Verification items for the finished model (mm, model axes). A direction names the side the tool comes from. Coordinates: 2 decimals unless noted, no trailing zeros. Loops run counter-clockwise (first coordinate to the right, second up) from the corner with the lowest first, then second, coordinate; pieces in that order, holes last.
Q1. Sectioned sample at B-B (z = 1.25). Count the separate pieces of the cut face and the enclosed holes in it, then the cut area to 3 significant figures.
Q2. Sectioned sample at A-A (y = 12.7). Enter the section's corners in (x, z).
Q3. Mould release check, pull along Y, two halves, no side actions. Record for faces 4 (the face through (-26.275, 12.83, 3.026)), 5 (the face through (0, -7, 6.35)), 6 (the face through (-1, -44.069, 3)): +Y half, -Y half, draft (parallel to the pull), parting line (faces both ways), or undercut.
Q4. Access from +Z, -Z, +X, -X, +Y, -Y to the whole of each face (thin tool, end or side, straight path). Record for faces 1 (the face through (15.594, -12.586, 6.162)), 2 (the face through (15.213, -12.806, 3.026)), 3 (the face through (-0.4, 19.2, 6.35)).
Q5. Sectioned sample at C-C (x = -23.5). Enter the section's corners in (y, z), then the cut area to 3 significant figures.
Q6. Go/stop test with flat-tipped pins: P1, Ø2.5, axis at x = -52.39, y = -39.69, coming from the -Z side; P2, Ø6.5, axis at x = -10, y = 15.5, coming from the +Z side. Record where each tip stops, or that it passes through.
Q7. Material ranges on probe 1 along Y at (x, z) = (10, 4); probe 2 along Y at (x, z) = (13.5, 1.25); probe 3 along X at (y, z) = (-17.5, 6.25), recorded low to high.
```python
from build123d import *

# Parameters (mm, degrees)
SKETCH1_W                 = 113.538
SKETCH1_H                 = 88.138
EXTRUDE1_DEPTH            = 6.35
F_8_CLEARANCE_HOLE1_D     = 4.0386
F_8_CLEARANCE_HOLE1_DEPTH = 6.35
FILLET2_R                 = 3.175
SKETCH8_W                 = 40.6908
SKETCH8_H                 = 12.6238
SKETCH8_W_2               = 20.7772
SKETCH8_H_2               = 10.414
CUT_EXTRUDE1_DEPTH        = 0.381
CUT_EXTRUDE2_DEPTH        = 7.35
CUT_EXTRUDE3_DEPTH        = 0.254


with BuildPart() as part:
    # Sketch1 → Extrude1 (new body)
    with BuildSketch(Plane.XY):
        Rectangle(SKETCH1_W, SKETCH1_H)
    extrude(amount=EXTRUDE1_DEPTH)

    # #8 Clearance Hole1
    with Locations(Plane(origin=(-52.3875, 39.6875, 6.35), x_dir=(1, 0, 0), z_dir=(0, 0, 1))):
        with Locations((0, 0), (104.775, 0), (104.775, -79.375), (0, -79.375)):
            Hole(F_8_CLEARANCE_HOLE1_D / 2, depth=F_8_CLEARANCE_HOLE1_DEPTH)

    # Fillet2
    fillet2_edges = [part.edges().sort_by_distance(p)[0] for p in [
        (-56.769, 44.069, 3.175),
        (56.769, 44.069, 3.175),
        (56.769, -44.069, 3.175),
        (-56.769, -44.069, 3.175),
    ]]
    fillet(fillet2_edges, radius=FILLET2_R)

    # Sketch8 → Cut-Extrude1 (cut)
    with BuildSketch(Plane.XY.offset(6.35)):
        with BuildLine():
            ThreePointArc((-20.3454, 6.3881), (-26.6573, 12.7), (-20.3454, 19.0119))
            Line((-20.3454, 19.0119), (-20.3454, 6.3881))
        make_face()
        with Locations((0, 12.7)):
            Rectangle(SKETCH8_W, SKETCH8_H)
        with BuildLine():
            ThreePointArc((20.3454, 19.0119), (26.6573, 12.7), (20.3454, 6.3881))
            Line((20.3454, 6.3881), (20.3454, 19.0119))
        make_face()
        with BuildLine():
            ThreePointArc((10.3886, -7.493), (15.5956, -12.7), (10.3886, -17.907))
            Line((10.3886, -17.907), (10.3886, -7.493))
        make_face()
        with Locations((0, -12.7)):
            Rectangle(SKETCH8_W_2, SKETCH8_H_2)
        with BuildLine():
            Line((-10.3886, -17.907), (-10.3886, -7.493))
            ThreePointArc((-10.3886, -7.493), (-15.5956, -12.7), (-10.3886, -17.907))
        make_face()
    extrude(amount=-CUT_EXTRUDE1_DEPTH, mode=Mode.SUBTRACT)

    # Sketch9 → Cut-Extrude2 (cut, through all)
    with BuildSketch(Plane.XY.offset(6.35)):
        with BuildLine():
            Line((-20.3454, 6.7691), (20.3454, 6.7691))
            ThreePointArc((20.3454, 6.7691), (26.2763, 12.7), (20.3454, 18.6309))
            Line((20.3454, 18.6309), (-20.3454, 18.6309))
            ThreePointArc((-20.3454, 18.6309), (-26.2763, 12.7), (-20.3454, 6.7691))
        make_face()
        with BuildLine():
            Line((10.3886, -7.874), (-10.3886, -7.874))
            ThreePointArc((-10.3886, -7.874), (-15.2146, -12.7), (-10.3886, -17.526))
            Line((-10.3886, -17.526), (10.3886, -17.526))
            ThreePointArc((10.3886, -17.526), (15.2146, -12.7), (10.3886, -7.874))
        make_face()
    extrude(amount=-CUT_EXTRUDE2_DEPTH, mode=Mode.SUBTRACT)

    # Sketch10 → Cut-Extrude3 (cut)
    with BuildSketch(Plane.XY.offset(6.35)):
        with BuildLine():
            Line((20.3454, 2.9591), (-20.3454, 2.9591))
            ThreePointArc((-20.3454, 2.9591), (-30.0863, 12.7), (-20.3454, 22.4409))
            Line((-20.3454, 22.4409), (20.3454, 22.4409))
            ThreePointArc((20.3454, 22.4409), (30.0863, 12.7), (20.3454, 2.9591))
        make_face()
        with BuildLine():
            ThreePointArc((20.3454, 3.2131), (29.8323, 12.7), (20.3454, 22.1869))
            Line((20.3454, 22.1869), (-20.3454, 22.1869))
            ThreePointArc((-20.3454, 22.1869), (-29.8323, 12.7), (-20.3454, 3.2131))
            Line((-20.3454, 3.2131), (20.3454, 3.2131))
        make_face(mode=Mode.SUBTRACT)
        with BuildLine():
            Line((10.3886, -21.336), (-10.3886, -21.336))
            ThreePointArc((-10.3886, -21.336), (-19.0246, -12.7), (-10.3886, -4.064))
            Line((-10.3886, -4.064), (10.3886, -4.064))
            ThreePointArc((10.3886, -4.064), (19.0246, -12.7), (10.3886, -21.336))
        make_face()
        with BuildLine():
            ThreePointArc((10.3886, -21.082), (18.7706, -12.7), (10.3886, -4.318))
            Line((10.3886, -4.318), (-10.3886, -4.318))
            ThreePointArc((-10.3886, -4.318), (-18.7706, -12.7), (-10.3886, -21.082))
            Line((-10.3886, -21.082), (10.3886, -21.082))
        make_face(mode=Mode.SUBTRACT)
    extrude(amount=-CUT_EXTRUDE3_DEPTH, mode=Mode.SUBTRACT)


solid = part.part
```
Geometry check:
1. separate pieces: 1
1. enclosed holes: 6
1. area: 9,080 mm2
2. outline: (-56.77, 0) - (-26.28, 0) - (-26.28, 5.97) - (-26.66, 5.97) - (-26.66, 6.35) - (-29.83, 6.35) - (-29.83, 6.1) - (-30.09, 6.1) - (-30.09, 6.35) - (-56.77, 6.35) - close; (26.28, 0) - (56.77, 0) - (56.77, 6.35) - (30.09, 6.35) - (30.09, 6.1) - (29.83, 6.1) - (29.83, 6.35) - (26.66, 6.35) - (26.66, 5.97) - (26.28, 5.97) - close
3. face 4: undercut
3. face 5: draft
3. face 6: -Y half
4. face 1: +Z
4. face 2: +Z, -Z
4. face 3: +Z, +X, -X, +Y, -Y
5. outline: (-44.07, 0) - (7.68, 0) - (7.68, 5.97) - (7.23, 5.97) - (7.23, 6.35) - (3.75, 6.35) - (3.75, 6.1) - (3.48, 6.1) - (3.48, 6.35) - (-44.07, 6.35) - close; (17.72, 0) - (44.07, 0) - (44.07, 6.35) - (21.92, 6.35) - (21.92, 6.1) - (21.65, 6.1) - (21.65, 6.35) - (18.17, 6.35) - (18.17, 5.97) - (17.72, 5.97) - close
5. area: 495 mm2
6. P1: passes through
6. P2: stops at z = 5.97
7. probe 1: y = -44.07 to -17.53, -7.87 to 6.77, 18.63 to 44.07
7. probe 2: y = -44.07 to -16.39, -9.01 to 6.77, 18.63 to 44.07
7. probe 3: x = -56.77 to -17.57, -17.26 to -12.41, 12.41 to 17.26, 17.57 to 56.77
